The model under review builds one solid part; all positions refer to its coordinate system, in mm. Face numbers are marked on the shaded views. A direction names the side the tool comes from. Coordinates: 2 decimals unless noted, no trailing zeros. One line per item, written item: value.
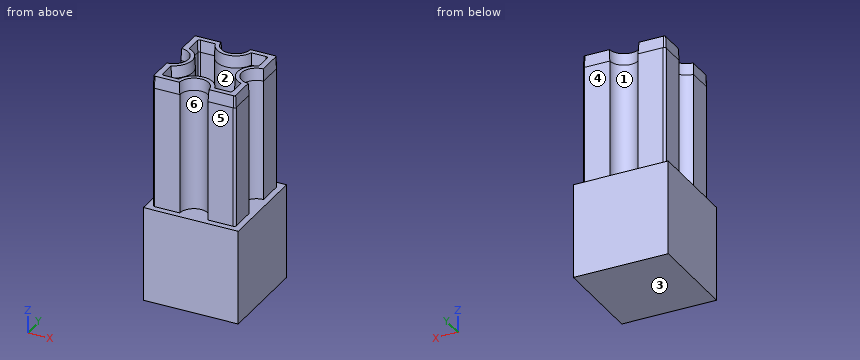
```python
from build123d import *

# Parameters (mm, degrees)
F0_W     = 23.5
F0_H     = 23.5
F1_DEPTH = 23.5
F3_DEPTH = 30
F4_DEPTH = 3
F4_TAPER = 3


with BuildPart() as f1:
    # F0 (on Top) → F1 (new body)
    with BuildSketch(Plane.XY):
        Rectangle(F0_W, F0_H)
    extrude(amount=F1_DEPTH)

    # F2 (on face) → F3 (join)
    with BuildSketch(Plane.XY.offset(23.5)):
        with BuildLine():
            ThreePointArc((3.5, 10.25), (0, 6.75), (-3.5, 10.25))
            Line((-3.5, 10.25), (-9.75, 10.25))
            ThreePointArc((-9.75, 10.25), (-10.1035533906, 10.1035533906), (-10.25, 9.75))
            Line((-10.25, 9.75), (-10.25, 3.5))
            ThreePointArc((-10.25, 3.5), (-6.75, 0), (-10.25, -3.5))
            Line((-10.25, -3.5), (-10.25, -9.75))
            ThreePointArc((-10.25, -9.75), (-10.1035533906, -10.1035533906), (-9.75, -10.25))
            Line((-9.75, -10.25), (-3.5, -10.25))
            ThreePointArc((-3.5, -10.25), (0, -6.75), (3.5, -10.25))
            Line((3.5, -10.25), (9.75, -10.25))
            ThreePointArc((9.75, -10.25), (10.1035533906, -10.1035533906), (10.25, -9.75))
            Line((10.25, -9.75), (10.25, -3.5))
            ThreePointArc((10.25, -3.5), (6.75, 0), (10.25, 3.5))
            Line((10.25, 3.5), (10.25, 9.75))
            ThreePointArc((10.25, 9.75), (10.1035533906, 10.1035533906), (9.75, 10.25))
            Line((9.75, 10.25), (3.5, 10.25))
        make_face()
        with BuildLine():
            Line((-8.5, -8.35), (-8.5, -4.4696196706))
            ThreePointArc((-8.5, -4.4696196706), (-5.45, 0), (-8.5, 4.4696196706))
            Line((-8.5, 4.4696196706), (-8.5, 8.35))
            ThreePointArc((-8.5, 8.35), (-8.3828427125, 8.6328427125), (-8.1, 8.75))
            Line((-8.1, 8.75), (-4.5596052461, 8.75))
            ThreePointArc((-4.5596052461, 8.75), (0, 5.45), (4.5596052461, 8.75))
            Line((4.5596052461, 8.75), (8.1, 8.75))
            ThreePointArc((8.1, 8.75), (8.3828427125, 8.6328427125), (8.5, 8.35))
            Line((8.5, 8.35), (8.5, 4.4696196706))
            ThreePointArc((8.5, 4.4696196706), (5.45, 0), (8.5, -4.4696196706))
            Line((8.5, -4.4696196706), (8.5, -8.35))
            ThreePointArc((8.5, -8.35), (8.3828427125, -8.6328427125), (8.1, -8.75))
            Line((8.1, -8.75), (4.5596052461, -8.75))
            ThreePointArc((4.5596052461, -8.75), (0, -5.45), (-4.5596052461, -8.75))
            Line((-4.5596052461, -8.75), (-8.1, -8.75))
            ThreePointArc((-8.1, -8.75), (-8.3828427125, -8.6328427125), (-8.5, -8.35))
        make_face(mode=Mode.SUBTRACT)
    extrude(amount=F3_DEPTH)

    # F3_face (on face) → F4 (join)
    with BuildSketch(Plane.XY.offset(53.5)):
        with BuildLine():
            ThreePointArc((3.5, 10.25), (0, 6.75), (-3.5, 10.25))
            Line((-3.5, 10.25), (-9.75, 10.25))
            ThreePointArc((-9.75, 10.25), (-10.1035533906, 10.1035533906), (-10.25, 9.75))
            Line((-10.25, 9.75), (-10.25, 3.5))
            ThreePointArc((-10.25, 3.5), (-6.75, 0), (-10.25, -3.5))
            Line((-10.25, -3.5), (-10.25, -9.75))
            ThreePointArc((-10.25, -9.75), (-10.1035533906, -10.1035533906), (-9.75, -10.25))
            Line((-9.75, -10.25), (-3.5, -10.25))
            ThreePointArc((-3.5, -10.25), (0, -6.75), (3.5, -10.25))
            Line((3.5, -10.25), (9.75, -10.25))
            ThreePointArc((9.75, -10.25), (10.1035533906, -10.1035533906), (10.25, -9.75))
            Line((10.25, -9.75), (10.25, -3.5))
            ThreePointArc((10.25, -3.5), (6.75, 0), (10.25, 3.5))
            Line((10.25, 3.5), (10.25, 9.75))
            ThreePointArc((10.25, 9.75), (10.1035533906, 10.1035533906), (9.75, 10.25))
            Line((9.75, 10.25), (3.5, 10.25))
        make_face()
        with BuildLine():
            Line((-4.5596052461, -8.75), (-8.1, -8.75))
            ThreePointArc((-8.1, -8.75), (-8.3828427125, -8.6328427125), (-8.5, -8.35))
            Line((-8.5, -8.35), (-8.5, -4.4696196706))
            ThreePointArc((-8.5, -4.4696196706), (-5.45, 0), (-8.5, 4.4696196706))
            Line((-8.5, 4.4696196706), (-8.5, 8.35))
            ThreePointArc((-8.5, 8.35), (-8.3828427125, 8.6328427125), (-8.1, 8.75))
            Line((-8.1, 8.75), (-4.5596052461, 8.75))
            ThreePointArc((-4.5596052461, 8.75), (0, 5.45), (4.5596052461, 8.75))
            Line((4.5596052461, 8.75), (8.1, 8.75))
            ThreePointArc((8.1, 8.75), (8.3828427125, 8.6328427125), (8.5, 8.35))
            Line((8.5, 8.35), (8.5, 4.4696196706))
            ThreePointArc((8.5, 4.4696196706), (5.45, 0), (8.5, -4.4696196706))
            Line((8.5, -4.4696196706), (8.5, -8.35))
            ThreePointArc((8.5, -8.35), (8.3828427125, -8.6328427125), (8.1, -8.75))
            Line((8.1, -8.75), (4.5596052461, -8.75))
            ThreePointArc((4.5596052461, -8.75), (0, -5.45), (-4.5596052461, -8.75))
        make_face(mode=Mode.SUBTRACT)
    extrude(amount=F4_DEPTH, taper=F4_TAPER)


solid = f1.part
```
(1) Insertion check: pin 1 Ø7 at (x, z) = (5.5, 34) entering from +Y; pin 2 Ø4 at (x, y) = (-8.5, 4.5) entering from +Z; pin 3 Ø1.9 at (y, z) = (-6.5, 32) entering from +X; pin 4 Ø5 at (x, z) = (6.5, 32) entering from -Y. Each pin has a flat end and moves straight along its axis. Give the tip position at first contact, or say it passes through.
Checks:
pin 1: y = 10.25
pin 2: z = 56.5
pin 3: x = 10.25
pin 4: y = -10.25
(2) Draft analysis for pull direction Y (two halves, no side actions). For the marked faces 1, 2 and 3, state which applies: pulls with the +Y half, pulls with the -Y half, needs draft (parallel to the pull), parting line crosses it, or undercut.
Checks:
face 1: pulls with the +Y half
face 2: undercut
face 3: needs draft
(3) To check wall thickness, follow L1, parallel to X at y = -4.75, z = 29.5; L2, parallel to Y at x = -8.25, z = 50; L3, parallel to X at y = -1.5, z = 39.5. State the ranges of each line that lie inside material, in increasing order. Write a range as [from, to].
Checks:
L1: [-10.25, -8.5], [8.5, 10.25]
L2: [-10.25, -8.72], [-4.36, -2.87], [2.87, 4.36], [8.72, 10.25]
L3: [-7.09, -5.69], [5.69, 7.09]
(4) Tool access review of the marked faces 4, 5 and 6: name each direction out of +Z, -Z, +X, -X, +Y, -Y from which nothing blocks a thin tool from reaching the whole face with its end or side.
Checks:
face 4: +Z, +X, -X, +Y
face 5: +Z, +X, -X, -Y
face 6: +Z, -Y
